```python
from build123d import *

# Parameters (mm, degrees)
ESQUISSE1_R        = 3.25
BOSS_EXTRU_1_DEPTH = 10
CONG_1_R           = 3
CONG_2_R           = 1


with BuildPart() as part:
    # Esquisse1 → Boss.-Extru.1 (new body)
    with BuildSketch(Plane.XY):
        with BuildLine():
            Line((11.588403104, 18.910210832), (11.588403104, 26.910210832))
            Line((11.588403104, 26.910210832), (-45.661596896, 26.910210832))
            Line((-45.661596896, 26.910210832), (-45.661596896, 18.910210832))
            ThreePointArc((-45.661596896, 18.910210832), (-43.972846395, 16.059772269), (-40.661596896, 16.171598045))
            Line((-40.661596896, 16.171598045), (-40.661596896, 13.171598045))
            Line((-40.661596896, 13.171598045), (-48.661596896, 13.171598045))
            Line((-48.661596896, 13.171598045), (-48.661596896, 19.910210832))
            Line((-48.661596896, 19.910210832), (-56.661596896, 19.910210832))
            Line((-56.661596896, 19.910210832), (-56.661596896, 22.910210832))
            Line((-56.661596896, 22.910210832), (-48.661596896, 22.910210832))
            Line((-48.661596896, 22.910210832), (-48.661596896, 30.910210832))
            Line((-48.661596896, 30.910210832), (23.588403104, 30.910210832))
            Line((23.588403104, 30.910210832), (23.588403104, 18.910210832))
            ThreePointArc((23.588403104, 18.910210832), (17.588403104, 12.910210832), (11.588403104, 18.910210832))
        make_face()
        with Locations((17.588403104, 18.910210832)):
            Circle(ESQUISSE1_R, mode=Mode.SUBTRACT)
    extrude(amount=BOSS_EXTRU_1_DEPTH)

    # Congé1
    cong_1_edges = [part.edges().sort_by_distance(p)[0] for p in [
        (-56.661596896, 21.410210832, 0),
        (-48.661596896, 30.910210832, 5),
        (23.588403104, 30.910210832, 5),
        (-45.661596896, 26.910210832, 5),
        (-48.661596896, 13.171598045, 5),
        (-56.661596896, 21.410210832, 10),
    ]]
    fillet(cong_1_edges, radius=CONG_1_R)

    # Congé2
    cong_2_edges = [part.edges().sort_by_distance(p)[0] for p in [
        (-40.661596896, 13.171598045, 5),
    ]]
    fillet(cong_2_edges, radius=CONG_2_R)


solid = part.part
```
The model under review builds one solid part; all positions refer to its coordinate system, in mm. A direction names the side the tool comes from. Round coordinates to 2 decimals unless told otherwise and drop trailing zeros. Order: outer loops, then holes, each group sorted by start corner. A loop starts at its lowest first (then second) coordinate and runs counter-clockwise, first axis right, second up. Notation, with made-up numbers: (27, 61.25) -> (65, 61.25) arc R21 cw to (65, 86.25) -> close; hole circle Ø11 at (-13, 62.25). An arc over 180 degrees is marked (long way). Use a Markdown table: item, result.
Q1. Tool access review of faces 4 (the flat face through (-44, 13.172, 5)), 5 (the flat face through (-48.662, 25, 5)), 6 (the cylindrical face through (-44.015, 16.083, 4.93)), 7 (the flat face through (11.588, 23, 5)): name each direction out of +Z, -Z, +X, -X, +Y, -Y from which nothing blocks a thin tool from reaching the whole face with its end or side.
Values:
| item | result |
|---|---|
| face 4 | +Z, -Z, -X, -Y |
| face 5 | +Z, -Z, -X, +Y |
| face 6 | +Z, -Z |
| face 7 | +Z, -Z, -Y |
Q2. For line 1 (X direction, y = 18.25, z = 1); line 2 (Y direction, x = -15, z = 2.5); line 3 (X direction, y = 27, z = 5), list the stretches that pass through material, from the lowest coordinate up.
Values:
| item | result |
|---|---|
| line 1 | x = -48.66 to -45.59, 11.62 to 14.41, 20.77 to 23.55 |
| line 2 | y = 26.91 to 30.91 |
| line 3 | x = -48.66 to 23.59 |
Q3. We need section A-A on y = 17.5. Write out the cut boundary in (x, z), then the cut area to 3 significant figures.
Values:
| item | result |
|---|---|
| outline | (-48.66, 0) -> (-45.34, 0) -> (-45.34, 10) -> (-48.66, 10) -> close; (11.76, 0) -> (14.66, 0) -> (14.66, 10) -> (11.76, 10) -> close; (20.52, 0) -> (23.42, 0) -> (23.42, 10) -> (20.52, 10) -> close |
| area | 91.3 mm^2 |
Q4. Clearance check with flat-ended pins moving along their axes: P1, Ø1.6, axis at y = 15, z = 3.5, coming from the +X side; P2, Ø1.2, axis at x = -43.5, z = 3, coming from the -Y side; P3, Ø2.5, axis at y = 25.5, z = 4, coming from the -X side. State where each tip first meets the part, or that it passes through.
Values:
| item | result |
|---|---|
| P1 | stops at x = 22.72 |
| P2 | stops at y = 13.17 |
| P3 | stops at x = -48.66 |
Q5. We need section C-C on x = -33. Write out the cut boundary in (y, z).
Values:
| item | result |
|---|---|
| outline | (26.91, 0) -> (30.91, 0) -> (30.91, 10) -> (26.91, 10) -> close |
Q6. Mouldability with a two-part tool opening along X and no side actions: class faces 1 (the cylindrical face through (-55.806, 21.431, 0.902)), 2 (the flat face through (-15, 26.91, 5)), 3 (the flat face through (-53, 22.91, 5)) as +X half, -X half, draft (parallel to the pull), parting line (faces both ways), or undercut.
Values:
| item | result |
|---|---|
| face 1 | -X half |
| face 2 | undercut |
| face 3 | draft |
Q7. We need section D-D on y = 21. Write out the cut boundary in (x, z), then the cut area to 3 significant figures.
Values:
| item | result |
|---|---|
| outline | (-56.66, 3) arc R3 ccw to (-53.66, 0) -> (-45.66, 0) -> (-45.66, 10) -> (-53.66, 10) arc R3 ccw to (-56.66, 7) -> close; (11.59, 0) -> (15.1, 0) -> (15.1, 10) -> (11.59, 10) -> close; (20.08, 0) -> (23.59, 0) -> (23.59, 10) -> (20.08, 10) -> close |
| area | 176 mm^2 |
Q8. We need section B-B on z = 5.25. Write out the cut boundary in (x, y).
Values:
| item | result |
|---|---|
| outline | (-56.66, 19.91) -> (-48.66, 19.91) -> (-48.66, 16.17) arc R3 ccw to (-45.66, 13.17) -> (-41.66, 13.17) arc R1 ccw to (-40.66, 14.17) -> (-40.66, 16.17) arc R3.25 cw to (-45.66, 18.91) -> (-45.66, 23.91) arc R3 cw to (-42.66, 26.91) -> (11.59, 26.91) -> (11.59, 18.91) arc R6 ccw to (23.59, 18.91) -> (23.59, 27.91) arc R3 ccw to (20.59, 30.91) -> (-45.66, 30.91) arc R3 ccw to (-48.66, 27.91) -> (-48.66, 22.91) -> (-56.66, 22.91) -> close; hole circle Ø6.5 at (17.59, 18.91) |
